Check sheet for the modelled part. Datum: model origin and axes. Units: mm. Face numbers are marked on the shaded views. A direction names the side the tool comes from. Give positions to 0.01 mm unless a question says otherwise; leave off trailing zeros. Loops run counter-clockwise (first coordinate to the right, second up) from the corner with the lowest first, then second, coordinate; pieces in that order, holes last.
```python
from build123d import *

# Parameters (mm, degrees)
SKETCH1_W                = 85
SKETCH1_H                = 85
BOSS_EXTRUDE1_DEPTH      = 7
FILLET1_R                = 4
SHELL1_T                 = -2
SHELL1_THICKNESS_2_DEPTH = 1
BOSS_EXTRUDE2_START      = 1
BOSS_EXTRUDE2_DEPTH      = 6
CIRPATTERN5_COUNT        = 4
SKETCH4_R                = 1.75
CUT_EXTRUDE1_DEPTH       = 61.510329697
MOVE_FACE1_BY            = 0.5
MOVE_FACE1_2_BY          = 0.5
MOVE_FACE1_3_BY          = 0.5
MOVE_FACE1_4_BY          = 0.5
MOVE_FACE1_5_BY          = 0.5
MOVE_FACE1_6_BY          = 0.5
MOVE_FACE1_7_BY          = 0.5
MOVE_FACE1_8_BY          = 0.5
MOVE_FACE1_9_BY          = 0.5
MOVE_FACE1_10_BY         = 0.5
MOVE_FACE1_11_BY         = 0.5
MOVE_FACE1_12_BY         = 0.5
EXTRUDE_THIN1_DEPTH      = 1.5
CIRPATTERN6_COUNT        = 4
SKETCH15_R               = 3.25
CUT_EXTRUDE5_DEPTH       = 2
EXTRUDE_THIN2_START      = -2
SKETCH16_R               = 2.25
SKETCH16_R_2             = 1.75
EXTRUDE_THIN2_DEPTH      = 2
SKETCH17_R               = 1.5
CUT_EXTRUDE6_DEPTH       = 61.702141643
SKETCH22_R               = 3
SKETCH22_R_2             = 1.5
BOSS_EXTRUDE5_DEPTH      = 3
CHAMFER2_SIZE            = 3


with BuildPart() as part:
    # Sketch1 → Boss-Extrude1 (new body)
    with BuildSketch(Plane.XY):
        Rectangle(SKETCH1_W, SKETCH1_H)
    extrude(amount=BOSS_EXTRUDE1_DEPTH)

    # Fillet1
    fillet1_edges = [part.edges().sort_by_distance(p)[0] for p in [
        (42.5, -42.5, 3.5),
        (-42.5, -42.5, 3.5),
        (-42.5, 42.5, 3.5),
        (42.5, 42.5, 3.5),
    ]]
    fillet(fillet1_edges, radius=FILLET1_R)

    # Shell1
    shell1_openings = [part.faces().sort_by_distance(p)[0] for p in [
        (0, 0, 7),
    ]]
    offset(amount=SHELL1_T, openings=shell1_openings, kind=Kind.INTERSECTION)

    # Shell1 thickness 2 face (on inner face of the shell) → Shell1 thickness 2 (cut)
    with BuildSketch(Plane(origin=(0, 0, 2), x_dir=(-1, 0, 0), z_dir=(0, 0, -1))):
        with BuildLine():
            ThreePointArc((40.5, -38.5), (39.914213562, -39.914213562), (38.5, -40.5))
            Line((38.5, -40.5), (-38.5, -40.5))
            ThreePointArc((-38.5, -40.5), (-39.914213562, -39.914213562), (-40.5, -38.5))
            Line((-40.5, -38.5), (-40.5, 38.5))
            ThreePointArc((-40.5, 38.5), (-39.914213562, 39.914213562), (-38.5, 40.5))
            Line((-38.5, 40.5), (38.5, 40.5))
            ThreePointArc((38.5, 40.5), (39.914213562, 39.914213562), (40.5, 38.5))
            Line((40.5, 38.5), (40.5, -38.5))
        make_face()
    extrude(amount=SHELL1_THICKNESS_2_DEPTH, mode=Mode.SUBTRACT)


with BuildPart() as body_2:
    # Sketch3 → Boss-Extrude2 (new body)
    with BuildSketch(Plane.XY.offset(BOSS_EXTRUDE2_START)):
        with BuildLine():
            Line((33.5, 38), (33.5, 42.5))
            Line((33.5, 42.5), (38, 42.5))
            ThreePointArc((38, 42.5), (41.181980515, 41.181980515), (42.5, 38))
            Line((42.5, 38), (42.5, 33.5))
            Line((42.5, 33.5), (38, 33.5))
            ThreePointArc((38, 33.5), (34.818019485, 34.818019485), (33.5, 38))
        make_face()
    extrude(amount=BOSS_EXTRUDE2_DEPTH)


with BuildPart() as cirpattern5_1:
    # CirPattern5: pattern copy
    add(body_2.part.rotate(Axis((0, 0, 0), (0, 0, 1)), 1 * 360 / CIRPATTERN5_COUNT))


with BuildPart() as cirpattern5_2:
    # CirPattern5: pattern copy
    add(body_2.part.rotate(Axis((0, 0, 0), (0, 0, 1)), 2 * 360 / CIRPATTERN5_COUNT))


with BuildPart() as cirpattern5_3:
    # CirPattern5: pattern copy
    add(body_2.part.rotate(Axis((0, 0, 0), (0, 0, 1)), 3 * 360 / CIRPATTERN5_COUNT))


with BuildPart() as part_1:
    add(part.part)

    # Combine1: union CirPattern5_1, body 2, CirPattern5_2, CirPattern5_3
    add(cirpattern5_1.part)
    add(body_2.part)
    add(cirpattern5_2.part)
    add(cirpattern5_3.part)

    # Sketch4 → Cut-Extrude1 (cut, through all)
    with BuildSketch(Plane.XY.offset(7)):
        with Locations((38, 38)):
            Circle(SKETCH4_R)
    cut_extrude1 = extrude(amount=-CUT_EXTRUDE1_DEPTH, mode=Mode.SUBTRACT)

    # Move Face1: a face moved outward by 0.5
    extrude(part_1.faces().sort_by_distance((-33.5, 39.25, 4))[0], amount=MOVE_FACE1_BY, dir=(1, 0, 0))

    # Move Face1 2: a curved face moved outward by 0.5
    add(Solid.thicken(part_1.faces().sort_by_distance((-34.818019485, 34.818019485, 4))[0], MOVE_FACE1_2_BY))

    # Move Face1 3: a face moved outward by 0.5
    extrude(part_1.faces().sort_by_distance((-39.25, 33.5, 4))[0], amount=MOVE_FACE1_3_BY, dir=(0, -1, 0))

    # Move Face1 4: a face moved outward by 0.5
    extrude(part_1.faces().sort_by_distance((-33.5, -39.25, 4))[0], amount=MOVE_FACE1_4_BY, dir=(1, 0, 0))

    # Move Face1 5: a face moved outward by 0.5
    extrude(part_1.faces().sort_by_distance((-39.25, -33.5, 4))[0], amount=MOVE_FACE1_5_BY, dir=(0, 1, 0))

    # Move Face1 6: a curved face moved outward by 0.5
    add(Solid.thicken(part_1.faces().sort_by_distance((-34.818019485, -34.818019485, 4))[0], MOVE_FACE1_6_BY))

    # Move Face1 7: a face moved outward by 0.5
    extrude(part_1.faces().sort_by_distance((33.5, -39.25, 4))[0], amount=MOVE_FACE1_7_BY, dir=(-1, 0, 0))

    # Move Face1 8: a curved face moved outward by 0.5
    add(Solid.thicken(part_1.faces().sort_by_distance((34.818019485, -34.818019485, 4))[0], MOVE_FACE1_8_BY))

    # Move Face1 9: a face moved outward by 0.5
    extrude(part_1.faces().sort_by_distance((39.25, -33.5, 4))[0], amount=MOVE_FACE1_9_BY, dir=(0, 1, 0))

    # Move Face1 10: a face moved outward by 0.5
    extrude(part_1.faces().sort_by_distance((39.25, 33.5, 4))[0], amount=MOVE_FACE1_10_BY, dir=(0, -1, 0))

    # Move Face1 11: a face moved outward by 0.5
    extrude(part_1.faces().sort_by_distance((33.5, 39.25, 4))[0], amount=MOVE_FACE1_11_BY, dir=(-1, 0, 0))

    # Move Face1 12: a curved face moved outward by 0.5
    add(Solid.thicken(part_1.faces().sort_by_distance((34.818019485, 34.818019485, 4))[0], MOVE_FACE1_12_BY))

    # Sketch7 → Extrude-Thin1 (add)
    with BuildSketch(Plane.XY.offset(7)):
        with BuildLine():
            Line((38, -34), (41.5, -34))
            Line((41.5, -34), (41.5, 34))
            Line((41.5, 34), (38, 34))
            ThreePointArc((38, 34), (35.171572875, 35.171572875), (34, 38))
            Line((34, 38), (34, 41.5))
            Line((34, 41.5), (-34, 41.5))
            Line((-34, 41.5), (-34, 38))
            ThreePointArc((-34, 38), (-35.171572875, 35.171572875), (-38, 34))
            Line((-38, 34), (-41.5, 34))
            Line((-41.5, 34), (-41.5, -34))
            Line((-41.5, -34), (-38, -34))
            ThreePointArc((-38, -34), (-35.171572875, -35.171572875), (-34, -38))
            Line((-34, -38), (-34, -41.5))
            Line((-34, -41.5), (34, -41.5))
            Line((34, -41.5), (34, -38))
            ThreePointArc((34, -38), (35.171572875, -35.171572875), (38, -34))
        make_face()
        with BuildLine():
            Line((38, -33), (40.5, -33))
            Line((40.5, -33), (40.5, 33))
            Line((40.5, 33), (38, 33))
            ThreePointArc((38, 33), (34.464466094, 34.464466094), (33, 38))
            Line((33, 38), (33, 40.5))
            Line((33, 40.5), (-33, 40.5))
            Line((-33, 40.5), (-33, 38))
            ThreePointArc((-33, 38), (-34.464466094, 34.464466094), (-38, 33))
            Line((-38, 33), (-40.5, 33))
            Line((-40.5, 33), (-40.5, -33))
            Line((-40.5, -33), (-38, -33))
            ThreePointArc((-38, -33), (-34.464466094, -34.464466094), (-33, -38))
            Line((-33, -38), (-33, -40.5))
            Line((-33, -40.5), (33, -40.5))
            Line((33, -40.5), (33, -38))
            ThreePointArc((33, -38), (34.464466094, -34.464466094), (38, -33))
        make_face(mode=Mode.SUBTRACT)
    extrude(amount=EXTRUDE_THIN1_DEPTH)

    # CirPattern6: Cut-Extrude1 ×4 about axis
    cirpattern6_axis = Axis((0, 0, 0), (0, 0, 1))
    for i in range(1, CIRPATTERN6_COUNT):
        add(cut_extrude1.rotate(cirpattern6_axis, i * 360 / CIRPATTERN6_COUNT), mode=Mode.SUBTRACT)

    # Sketch15 → Cut-Extrude5 (cut)
    with BuildSketch(Plane(origin=(0, 0, 0), x_dir=(-1, 0, 0), z_dir=(0, 0, -1))):
        with Locations((-38, -38)):
            Circle(SKETCH15_R)
        with Locations((38, -38)):
            Circle(SKETCH15_R)
        with Locations((38, 38)):
            Circle(SKETCH15_R)
        with Locations((-38, 38)):
            Circle(SKETCH15_R)
    extrude(amount=-CUT_EXTRUDE5_DEPTH, mode=Mode.SUBTRACT)

    # Sketch16 → Extrude-Thin2 (add)
    # profile 1 of 4: a face of its own
    with BuildSketch(Plane(origin=(0, 0, 0), x_dir=(-1, 0, 0), z_dir=(0, 0, -1)).offset(EXTRUDE_THIN2_START)):
        with Locations((-38, -38)):
            Circle(SKETCH16_R)
        with Locations((-38, -38)):
            Circle(SKETCH16_R_2, mode=Mode.SUBTRACT)
    # profile 2 of 4: a face of its own
    with BuildSketch(Plane(origin=(0, 0, 0), x_dir=(-1, 0, 0), z_dir=(0, 0, -1)).offset(EXTRUDE_THIN2_START)):
        with Locations((-38, 38)):
            Circle(SKETCH16_R)
        with Locations((-38, 38)):
            Circle(SKETCH16_R_2, mode=Mode.SUBTRACT)
    # profile 3 of 4: a face of its own
    with BuildSketch(Plane(origin=(0, 0, 0), x_dir=(-1, 0, 0), z_dir=(0, 0, -1)).offset(EXTRUDE_THIN2_START)):
        with Locations((38, -38)):
            Circle(SKETCH16_R)
        with Locations((38, -38)):
            Circle(SKETCH16_R_2, mode=Mode.SUBTRACT)
    # profile 4 of 4: a face of its own
    with BuildSketch(Plane(origin=(0, 0, 0), x_dir=(-1, 0, 0), z_dir=(0, 0, -1)).offset(EXTRUDE_THIN2_START)):
        with Locations((38, 38)):
            Circle(SKETCH16_R)
        with Locations((38, 38)):
            Circle(SKETCH16_R_2, mode=Mode.SUBTRACT)
    extrude(amount=EXTRUDE_THIN2_DEPTH)

    # Sketch17 → Cut-Extrude6 (cut, through all)
    with BuildSketch(Plane(origin=(0, 0, 0), x_dir=(-1, 0, 0), z_dir=(0, 0, -1))):
        with Locations((0, -32.5)):
            Circle(SKETCH17_R)
    extrude(amount=-CUT_EXTRUDE6_DEPTH, mode=Mode.SUBTRACT)

    # Sketch22 → Boss-Extrude5 (add)
    with BuildSketch(Plane.XY.offset(1)):
        with Locations(Location((0, -32.5, 0), (0, 0, 180))):
            Circle(SKETCH22_R)
        with Locations(Location((0, -32.5, 0), (0, 0, 180))):
            Circle(SKETCH22_R_2, mode=Mode.SUBTRACT)
    extrude(amount=BOSS_EXTRUDE5_DEPTH)

    # Chamfer2
    chamfer2_edges = [part_1.edges().sort_by_distance(p)[0] for p in [
        (3, -32.5, 1),
    ]]
    chamfer(chamfer2_edges, length=CHAMFER2_SIZE - 0.0001)  # a hair under: the kernel refuses the full size


solid = part_1.part
```
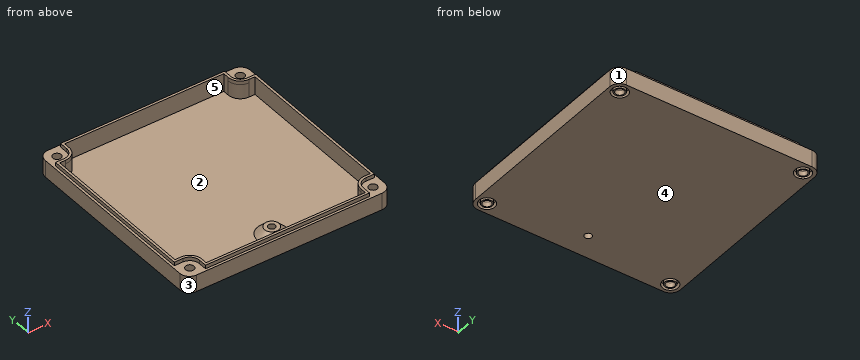
(1) Section check C-C on y = 26. Record the boundary of the cut face in (x, z), plus the area to 3 significant figures.
(2) Release check for a two-part mould opening along Y. For the marked faces 1, 2 and 3 record: pulls with the +Y half, pulls with the -Y half, needs draft (parallel to the pull), parting line crosses it, or undercut.
(3) Gauge pin test, flat ends, axial feed: pin 1 Ø4.5 at (x, y) = (38, 38) entering from +Z; pin 2 Ø1.2 at (y, z) = (40, 5) entering from -X; pin 3 Ø0.8 at (y, z) = (3.5, 8) entering from +X. Record the tip position at first contact, or that the pin passes through.
(4) Access from +Z, -Z, +X, -X, +Y, -Y to the whole of each face (thin tool, end or side, straight path). Record for the marked faces 4 and 5.
(5) Material ranges on line 1 (Y direction, x = 38, z = 5.1); line 2 (X direction, y = 29, z = 6.5); line 3 (Y direction, x = 0, z = 1.5), recorded low to high.
(6) Section check A-A on z = 5.5. Record the boundary of the cut face in (x, y), plus the area to 3 significant figures.
Computed values:
1. outline: (-42.5, 0) - (42.5, 0) - (42.5, 7) - (41.5, 7) - (41.5, 8.5) - (40.5, 8.5) - (40.5, 1) - (-40.5, 1) - (-40.5, 8.5) - (-41.5, 8.5) - (-41.5, 7) - (-42.5, 7) - close
1. area: 112 mm2
2. face 1: pulls with the +Y half
2. face 2: undercut
2. face 3: pulls with the -Y half
3. pin 1: stops at z = 7
3. pin 2: stops at x = -42.4
3. pin 3: stops at x = 41.5
4. face 4: -Z, +X, -X, +Y, -Y
4. face 5: +Z
5. line 1: y = -42.5 to -39.75, -36.25 to -33, 33 to 36.25, 39.75 to 42.5
5. line 2: x = -42.5 to -40.5, 40.5 to 42.5
5. line 3: y = -42.5 to -40.5, -38 to -34, -31 to -27, 40.5 to 42.5
6. outline: (-42.5, -38.5) arc R4 ccw to (-38.5, -42.5) - (38.5, -42.5) arc R4 ccw to (42.5, -38.5) - (42.5, 38.5) arc R4 ccw to (38.5, 42.5) - (-38.5, 42.5) arc R4 ccw to (-42.5, 38.5) - close; hole (-40.5, -33) - (-38, -33) arc R5 cw to (-33, -38) - (-33, -40.5) - (33, -40.5) - (33, -38) arc R5 cw to (38, -33) - (40.5, -33) - (40.5, 33) - (38, 33) arc R5 cw to (33, 38) - (33, 40.5) - (-33, 40.5) - (-33, 38) arc R5 cw to (-38, 33) - (-40.5, 33) - close; hole circle Ø3.5 at (-38, -38); hole circle Ø3.5 at (-38, 38); hole circle Ø3.5 at (38, -38); hole circle Ø3.5 at (38, 38)
6. area: 815 mm2
